```python
from build123d import *

# Parameters (mm, degrees)
CYLINDER005_R     = 1.8
CYLINDER005_DEPTH = 10
BOX010_W          = 8
BOX010_H          = 22
BOX010_DEPTH      = 3
CYLINDER009_R     = 1.5
CYLINDER009_DEPTH = 10
CYLINDER008_R     = 1.5
CYLINDER008_DEPTH = 10
CYLINDER007_R     = 1.5
CYLINDER007_DEPTH = 10
CYLINDER006_R     = 1.5
CYLINDER006_DEPTH = 10
BOX009_W          = 18
BOX009_H          = 18
BOX009_DEPTH      = 3


with BuildPart() as cylinder005:
    # Cylinder005 → Cylinder005 (new body)
    with BuildSketch(Plane(origin=(5, 2, 0), x_dir=(1, 0, 0), z_dir=(0, 0, 1))):
        Circle(CYLINDER005_R)
    extrude(amount=CYLINDER005_DEPTH)


with BuildPart() as cut012:
    # Box010 → Box010 (new body)
    with BuildSketch(Plane(origin=(1, -1, 0), x_dir=(1, 0, 0), z_dir=(0, 0, 1))):
        with Locations((4, 11)):
            Rectangle(BOX010_W, BOX010_H)
    extrude(amount=BOX010_DEPTH)

    # Cut012: cut Cylinder005
    add(cylinder005.part, mode=Mode.SUBTRACT)


with BuildPart() as cylinder009:
    # Cylinder009 → Cylinder009 (new body)
    with BuildSketch(Plane(origin=(5, 23.65, 0), x_dir=(1, 0, 0), z_dir=(0, 0, 1))):
        Circle(CYLINDER009_R)
    extrude(amount=CYLINDER009_DEPTH)


with BuildPart() as cylinder008:
    # Cylinder008 → Cylinder008 (new body)
    with BuildSketch(Plane(origin=(-1.35, 30, 0), x_dir=(1, 0, 0), z_dir=(0, 0, 1))):
        Circle(CYLINDER008_R)
    extrude(amount=CYLINDER008_DEPTH)


with BuildPart() as cylinder007:
    # Cylinder007 → Cylinder007 (new body)
    with BuildSketch(Plane(origin=(11.35, 30, 0), x_dir=(1, 0, 0), z_dir=(0, 0, 1))):
        Circle(CYLINDER007_R)
    extrude(amount=CYLINDER007_DEPTH)


with BuildPart() as cylinder006:
    # Cylinder006 → Cylinder006 (new body)
    with BuildSketch(Plane(origin=(5, 36.35, 0), x_dir=(1, 0, 0), z_dir=(0, 0, 1))):
        Circle(CYLINDER006_R)
    extrude(amount=CYLINDER006_DEPTH)


with BuildPart() as obj1:
    # Box009 → Box009 (new body)
    with BuildSketch(Plane(origin=(-4, 21, 0), x_dir=(1, 0, 0), z_dir=(0, 0, 1))):
        with Locations((9, 9)):
            Rectangle(BOX009_W, BOX009_H)
    extrude(amount=BOX009_DEPTH)

    # Cut008: cut Cylinder006
    add(cylinder006.part, mode=Mode.SUBTRACT)

    # Cut009: cut Cylinder007
    add(cylinder007.part, mode=Mode.SUBTRACT)

    # Cut010: cut Cylinder008
    add(cylinder008.part, mode=Mode.SUBTRACT)

    # Cut011: cut Cylinder009
    add(cylinder009.part, mode=Mode.SUBTRACT)

    # Fusion002: union Cut012
    add(cut012.part)


solid = obj1.part
```
Work out the finished part from the listing and answer in its coordinate system (mm). A direction names the side the tool comes from. Coordinates: 2 decimals unless noted, no trailing zeros. Loops run counter-clockwise (first coordinate to the right, second up) from the corner with the lowest first, then second, coordinate; pieces in that order, holes last.
1) Section A-A (z = 0.7) is taken. Give the vertices of the cut face in (x, y).
Results:
outline: (-4, 21) - (1, 21) - (1, -1) - (9, -1) - (9, 21) - (14, 21) - (14, 39) - (-4, 39) - close; hole circle Ø3 at (-1.35, 30); hole circle Ø3.6 at (5, 2); hole circle Ø3 at (5, 23.65); hole circle Ø3 at (5, 36.35); hole circle Ø3 at (11.35, 30)
2) Section B-B (y = 36.35) is taken. Give the vertices of the cut face in (x, z).
Results:
outline: (-4, 0) - (3.5, 0) - (3.5, 3) - (-4, 3) - close; (6.5, 0) - (14, 0) - (14, 3) - (6.5, 3) - close
3) Consider probe 1 along Y at (x, z) = (5, 1.35); probe 2 along X at (y, z) = (30, 1.05); probe 3 along Y at (x, z) = (11.5, 0.25). Determine where each line is inside the solid, lowest interval first.
Results:
probe 1: y = -1 to 0.2, 3.8 to 22.15, 25.15 to 34.85, 37.85 to 39
probe 2: x = -4 to -2.85, 0.15 to 9.85, 12.85 to 14
probe 3: y = 21 to 28.51, 31.49 to 39
4) For faces 4 (the cylindrical face through (6.43, 36.8, 1.48)), 5 (the flat face through (1, 10, 1)), 6 (the flat face through (11, 21, 1)), determine the directions among +Z, -Z, +X, -X, +Y, -Y from which every point of the face is accessible in a straight line to the end or side of a thin tool.
Results:
face 4: +Z, -Z
face 5: +Z, -Z, -X, -Y
face 6: +Z, -Z, +X, -Y
5) Section C-C (x = 5) is taken. Give the vertices of the cut face in (y, z), plus the area to 3 significant figures.
Results:
outline: (-1, 0) - (0.2, 0) - (0.2, 3) - (-1, 3) - close; (3.8, 0) - (22.15, 0) - (22.15, 3) - (3.8, 3) - close; (25.15, 0) - (34.85, 0) - (34.85, 3) - (25.15, 3) - close; (37.85, 0) - (39, 0) - (39, 3) - (37.85, 3) - close
area: 91.2 mm2
6) For a pull along X with two mould halves and no side action, classify faces 1 (the flat face through (-2, 21, 1)), 2 (the flat face through (9, 10, 1)), 3 (the cylindrical face through (11.155, 31.487, 1.479)) as +X half, -X half, draft (parallel to the pull), parting line (faces both ways), or undercut.
Results:
face 1: draft
face 2: +X half
face 3: undercut
7) Section D-D (x = 11) is taken. Give the vertices of the cut face in (y, z).
Results:
outline: (21, 0) - (28.54, 0) - (28.54, 3) - (21, 3) - close; (31.46, 0) - (39, 0) - (39, 3) - (31.46, 3) - close
8) Flat-ended cylindrical pins translate along their axes: pin 1 (3 mm diameter, centred on x = 5, y = 2, fed in from -Z); pin 2 (0.9 mm diameter, centred on y = 10.5, z = 1.5, fed in from -X). Find the tip coordinate at first contact, or state that the pin passes through.
Results:
pin 1: passes through
pin 2: stops at x = 1
